```python
from build123d import *

# Parameters (mm, degrees)
F1_DEPTH = 20
F3_D     = 9
F5_D     = 9
F7_D     = 4.2


with BuildPart() as f1:
    # F0 (on Front) → F1 (new body)
    with BuildSketch(Plane.XZ):
        Polygon((0, 104), (0, 0), (-16, 0), (-16, -10), (0, -10), (0, -35), (10, -35), (10, 104), align=None)
    extrude(amount=F1_DEPTH)

    # F3 (through all)
    with Locations(Plane.XY):
        with Locations((-8, -10)):
            Hole(F3_D / 2)

    # F5 (through all)
    with Locations(Plane.YZ.offset(10)):
        with Locations((-10, -28)):
            Hole(F5_D / 2)

    # F7 (through all)
    with Locations(Plane.YZ.offset(10)):
        with Locations((-10, 97.5), (-10, 5.5)):
            Hole(F7_D / 2)


solid = f1.part
```
CAD build for the part. Positions are in the model's coordinates, mm. A direction names the side the tool comes from. Coordinates: 2 decimals unless noted, no trailing zeros. Loops run counter-clockwise (first coordinate to the right, second up) from the corner with the lowest first, then second, coordinate; pieces in that order, holes last. Notation, with made-up numbers: (-39, 33.5) - (-11, 33.5) arc R12 ccw to (-11, 48.5) - close; hole circle Ø4 at (-25, -2). An arc over 180 degrees is marked (long way). Return JSON: item names as keys, results as strings.
1. Drop flat-ended pins along their axis: pin 1 (1 mm diameter, centred on x = -5, y = -13, fed in from +Z); pin 2 (2 mm diameter, centred on y = -16, z = -15.5, fed in from -X); pin 3 (5 mm diameter, centred on x = -6.5, y = -2.5, fed in from -Z); pin 4 (2.5 mm diameter, centred on y = -10, z = 97.5, fed in from -X). Give the stop position or say it passes through.
Result:
{"pin 1": "stops at z = 0", "pin 2": "stops at x = 0", "pin 3": "stops at z = -10", "pin 4": "passes through"}
2. Band-saw the part on D-D (x = 6.25). Give the cut face in (y, z), and give its area (3 significant figures).
Result:
{"outline": "(-20, -35) - (0, -35) - (0, 104) - (-20, 104) - close; hole circle Ø9 at (-10, -28); hole circle Ø4.2 at (-10, 5.5); hole circle Ø4.2 at (-10, 97.5)", "area": "2,690 mm2"}
3. Band-saw the part on B-B (z = 5.5). Give the cut face in (x, y).
Result:
{"outline": "(0, -20) - (10, -20) - (10, -12.1) - (0, -12.1) - close; (0, -7.9) - (10, -7.9) - (10, 0) - (0, 0) - close"}
4. Mould opens along Y. For faces 1 (the flat face through (5, -20, 25)), 2 (the cylindrical face through (4.93, -8.452, 6.919)), 3 (the cylindrical face through (4.93, -14.292, -26.648)), 4 (the flat face through (5, -10, 104)) say: released by +Y, released by -Y, zero draft, split by the parting line, or undercut.
Result:
{"face 1": "released by -Y", "face 2": "undercut", "face 3": "undercut", "face 4": "zero draft"}
5. 3-axis set-ups, long thin cutter, end or side, ignore diameter. For faces 5 (the flat face through (0, -10, -22)), 6 (the flat face through (-8, -5, 0)), 7 (the cylindrical face through (4.93, -8.334, 96.222)): which of +Z, -Z, +X, -X, +Y, -Y reach the whole face in a straight line?
Result:
{"face 5": "-Z, -X, +Y, -Y", "face 6": "+Z, -X, +Y, -Y", "face 7": "+X, -X"}
6. Band-saw the part on C-C (x = -8). Give the cut face in (y, z).
Result:
{"outline": "(-20, -10) - (-14.5, -10) - (-14.5, 0) - (-20, 0) - close; (-5.5, -10) - (0, -10) - (0, 0) - (-5.5, 0) - close"}
7. Probe L1, parallel to Z at x = 2, y = -10; L2, parallel to Y at x = -8, z = -3.5; L3, parallel to Z at x = 1.5, y = -11.75. List the from-to ranges inside material, lowest first. Write a range as from..to.
Result:
{"L1": "z = -35..-32.5, -23.5..3.4, 7.6..95.4, 99.6..104", "L2": "y = -20..-14.5, -5.5..0", "L3": "z = -35..-32.15, -23.85..4.34, 6.66..96.34, 98.66..104"}
8. Band-saw the part on A-A (y = -10). Give the cut face in (x, z), and give its area (3 significant figures).
Result:
{"outline": "(-16, -10) - (-12.5, -10) - (-12.5, 0) - (-16, 0) - close; (-3.5, -10) - (0, -10) - (0, -23.5) - (10, -23.5) - (10, 3.4) - (0, 3.4) - (0, 0) - (-3.5, 0) - close; (0, -35) - (10, -35) - (10, -32.5) - (0, -32.5) - close; (0, 7.6) - (10, 7.6) - (10, 95.4) - (0, 95.4) - close; (0, 99.6) - (10, 99.6) - (10, 104) - (0, 104) - close", "area": "1,290 mm2"}
